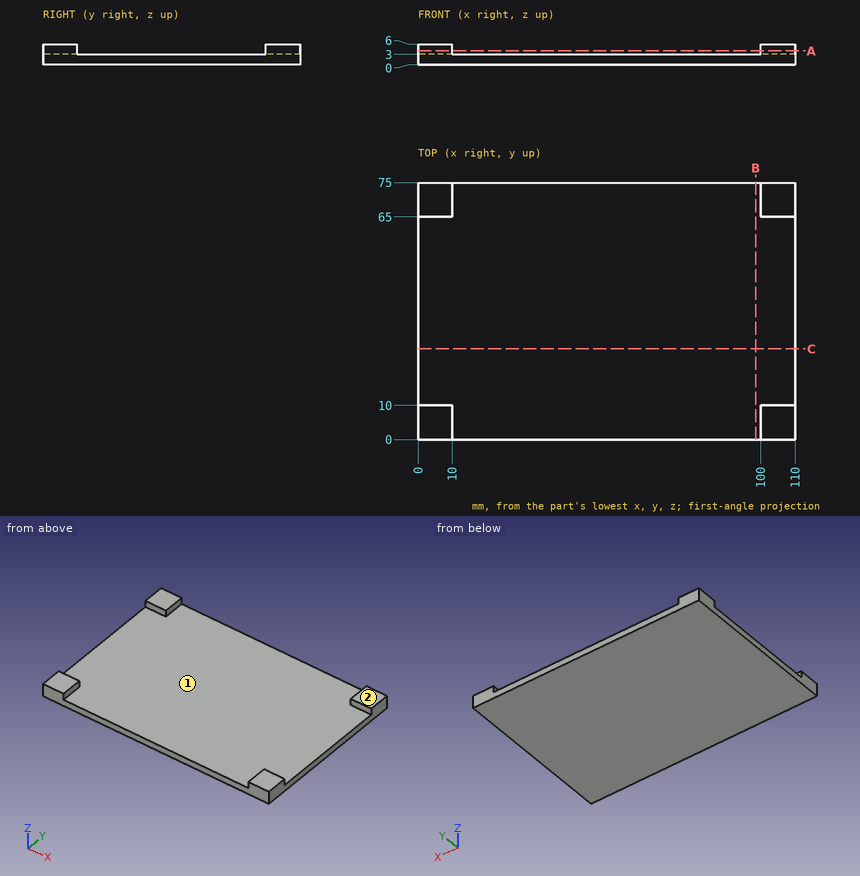
Check sheet for the drawn part. Datum: minimum x, y, z corner. Units: mm. Coordinates: 2 decimals unless noted, no trailing zeros. Order: outer loops, then holes, each group sorted by start corner. A loop starts at its lowest first (then second) coordinate and runs counter-clockwise, first axis right, second up. Notation, with made-up numbers: (-26.5, 70.25) -> (9.5, 70.25) arc R22 cw to (9.5, 92.25) -> close; hole circle Ø10 at (47.25, -25). An arc over 180 degrees is marked (long way). Write each question's results on one line, items separated by ' | '. Start each with the question number.
1) Section check A-A (z = 4). Enter the section's corners in (x, y).
2) Section check C-C (y = 26.5). Enter the section's corners in (x, z), and give its area (3 significant figures).
3) Draft check along X on the marked faces 1 and 2. Enter one of: pulls with the +X half, pulls with the -X half, needs draft (parallel to the pull), parting line crosses it, or undercut.
4) Depth check by flat-ended pin: pin 1 (12 mm diameter, centred on x = 20.5, y = 38, fed in from +Z). Enter the tip coordinate at first touch or a pass-through.
5) Section check B-B (x = 98.5). Enter the section's corners in (y, z), and give its area (3 significant figures).
6) Material ranges on line 1 along X through (y, z) = (4, 4.15); line 2 along Z through (x, y) = (59.5, 46.5), recorded low to high.
Checked values:
1) outline: (0, 0) -> (10, 0) -> (10, 10) -> (0, 10) -> close; (0, 65) -> (10, 65) -> (10, 75) -> (0, 75) -> close; (100, 0) -> (110, 0) -> (110, 10) -> (100, 10) -> close; (100, 65) -> (110, 65) -> (110, 75) -> (100, 75) -> close
2) outline: (0, 0) -> (110, 0) -> (110, 3) -> (0, 3) -> close | area: 330 mm²
3) face 1: undercut | face 2: needs draft
4) pin 1: z = 3
5) outline: (0, 0) -> (75, 0) -> (75, 3) -> (0, 3) -> close | area: 225 mm²
6) line 1: 0 to 10, 100 to 110 | line 2: 0 to 3
